CAD build for the part. Positions are in the model's coordinates, mm. Round coordinates to 2 decimals unless told otherwise and drop trailing zeros. Write each loop counter-clockwise with the first axis right and the second up, starting at its lowest first coordinate (ties: lowest second). Pieces come first, ordered by that corner, then holes. Notation, with made-up numbers: (34.5, -19) -> (64.5, -19) arc R32 cw to (64.5, 12) -> close; hole circle Ø3 at (45.25, 34). An arc over 180 degrees is marked (long way). Answer in a Markdown table with one row per item. Add a question column.
```python
from build123d import *

# Parameters (mm, degrees)
SKETCH1_W           = 66
SKETCH1_H           = 50
SKETCH1_R           = 1
BOSS_EXTRUDE1_DEPTH = 5
SKETCH2_R           = 1
CUT_EXTRUDE1_DEPTH  = 388.996134001
SKETCH3_R           = 1
SKETCH3_W           = 20
SKETCH3_H           = 5
CUT_EXTRUDE2_DEPTH  = 388.996134001
CUT_EXTRUDE3_DEPTH  = 388.996134001
SKETCH5_OUTSIDE_W   = 171.322
SKETCH5_OUTSIDE_H   = 295.322
SKETCH5_OUTSIDE_W_2 = 29
SKETCH5_OUTSIDE_H_2 = 26.5
CUT_EXTRUDE4_DEPTH  = 388.996134001


with BuildPart() as part:
    # Sketch1 → Boss-Extrude1 (new body)
    # profile 1 of 3: a face of its own
    with BuildSketch(Plane.XY):
        with Locations((-33, 85)):
            Rectangle(SKETCH1_W, SKETCH1_H)
    # profile 2 of 3: a face of its own
    with BuildSketch(Plane.XY):
        Polygon((0, 60), (0, 0), (180, 0), (180, 60), (180, 110), (180, 300), (130, 300), (130, 150), (50, 150), (50, 300), (0, 300), (0, 110), align=None)
        with Locations((19, 117.5)):
            Circle(SKETCH1_R, mode=Mode.SUBTRACT)
        with Locations((38, 117.5)):
            Circle(SKETCH1_R, mode=Mode.SUBTRACT)
        with Locations((19, 134)):
            Circle(SKETCH1_R, mode=Mode.SUBTRACT)
        with Locations((38, 134)):
            Circle(SKETCH1_R, mode=Mode.SUBTRACT)
        with Locations((142, 117.5)):
            Circle(SKETCH1_R, mode=Mode.SUBTRACT)
        with Locations((161, 117.5)):
            Circle(SKETCH1_R, mode=Mode.SUBTRACT)
        with Locations((142, 134)):
            Circle(SKETCH1_R, mode=Mode.SUBTRACT)
        with Locations((161, 134)):
            Circle(SKETCH1_R, mode=Mode.SUBTRACT)
    # profile 3 of 3: a face of its own
    with BuildSketch(Plane.XY):
        with Locations((213, 85)):
            Rectangle(SKETCH1_W, SKETCH1_H)
    extrude(amount=BOSS_EXTRUDE1_DEPTH)

    # Sketch2 → Cut-Extrude1 (cut, through all)
    with BuildSketch(Plane.XY.offset(5)):
        with Locations((-58, 103)):
            Circle(SKETCH2_R)
        with Locations((-58, 67)):
            Circle(SKETCH2_R)
        with Locations(Location((238, 67, 0), (0, 0, 180))):
            Circle(SKETCH2_R)
        with Locations(Location((238, 103, 0), (0, 0, 180))):
            Circle(SKETCH2_R)
    extrude(amount=-CUT_EXTRUDE1_DEPTH, mode=Mode.SUBTRACT)

    # Sketch3 → Cut-Extrude2 (cut, through all)
    with BuildSketch(Plane.XY.offset(5)):
        with Locations((19, 77)):
            Circle(SKETCH3_R)
        with Locations((19, 99.5)):
            Circle(SKETCH3_R)
        with Locations(Location((161, 77, 0), (0, 0, 180))):
            Circle(SKETCH3_R)
        with Locations(Location((161, 99.5, 0), (0, 0, 180))):
            Circle(SKETCH3_R)
        with Locations((-6, 90)):
            Rectangle(SKETCH3_W, SKETCH3_H)
        with Locations((186, 90)):
            Rectangle(SKETCH3_W, SKETCH3_H)
    extrude(amount=-CUT_EXTRUDE2_DEPTH, mode=Mode.SUBTRACT)

    # Sketch4 → Cut-Extrude3 (cut, through all)
    with BuildSketch(Plane.XY.offset(5)):
        Polygon((180, 60), (130, 60), (130, 150), (65.062754068, 311.897276324), (-51.051297303, 321.248743549), (-107.939389585, -9.16976505), (175.332138424, -20.859099081), (198.321162017, 8.753880463), align=None)
    extrude(amount=-CUT_EXTRUDE3_DEPTH, mode=Mode.SUBTRACT)

    # Sketch5 outside → Cut-Extrude4 (cut, through all)
    with BuildSketch(Plane(origin=(0, 0, 0), x_dir=(-1, 0, 0), z_dir=(0, 0, -1))):
        with Locations((-188, 180)):
            Rectangle(SKETCH5_OUTSIDE_W, SKETCH5_OUTSIDE_H)
        with Locations((-151.5, 125.75)):
            Rectangle(SKETCH5_OUTSIDE_W_2, SKETCH5_OUTSIDE_H_2, mode=Mode.SUBTRACT)
    extrude(amount=-CUT_EXTRUDE4_DEPTH, mode=Mode.SUBTRACT)


solid = part.part
```
Item 1: Saw through at B-B on x = 161. Give the cut face in (y, z), then the cut area to 4 significant figures.
Item 2: Saw through at C-C on z = 2.8. Give the cut face in (x, y).
Item 3: Saw through at A-A on y = 117.5. Give the cut face in (x, z), then the cut area to 3 significant figures.
Item 4: Pin check, flat tip, straight feed: pin 1 (1.8 mm diameter, centred on x = 142, y = 117.5, fed in from -Z). Stop position of the tip, or through.
Item 5: Two-plate mould, pull along Y, no slides. Class faces 1 (the flat face through (151, 126, 0)), 2 (the flat face through (152, 139, 2)), 3 (the cylindrical face through (160.2, 116.9, 2.5)): +Y half, -Y half, draft (parallel to the pull), parting line (faces both ways), or undercut.
Item 6: Drill centre lines: probe 1 along Y at (x, z) = (142, 2.45); probe 2 along Y at (x, z) = (142.5, 0.55). Where is each one in solid material? Low to high.
Recorded:
| question | item | result |
|---|---|---|
| 1 | outline | (112.5, 0) -> (116.5, 0) -> (116.5, 5) -> (112.5, 5) -> close; (118.5, 0) -> (133, 0) -> (133, 5) -> (118.5, 5) -> close; (135, 0) -> (139, 0) -> (139, 5) -> (135, 5) -> close |
| 1 | area | 112.5 mm2 |
| 2 | outline | (137, 112.5) -> (166, 112.5) -> (166, 139) -> (137, 139) -> close; hole circle Ø2 at (142, 117.5); hole circle Ø2 at (142, 134); hole circle Ø2 at (161, 117.5); hole circle Ø2 at (161, 134) |
| 3 | outline | (137, 0) -> (141, 0) -> (141, 5) -> (137, 5) -> close; (143, 0) -> (160, 0) -> (160, 5) -> (143, 5) -> close; (162, 0) -> (166, 0) -> (166, 5) -> (162, 5) -> close |
| 3 | area | 125 mm2 |
| 4 | pin 1 | through |
| 5 | face 1 | draft |
| 5 | face 2 | +Y half |
| 5 | face 3 | undercut |
| 6 | probe 1 | 112.5 to 116.5, 118.5 to 133, 135 to 139 |
| 6 | probe 2 | 112.5 to 116.63, 118.37 to 133.13, 134.87 to 139 |
